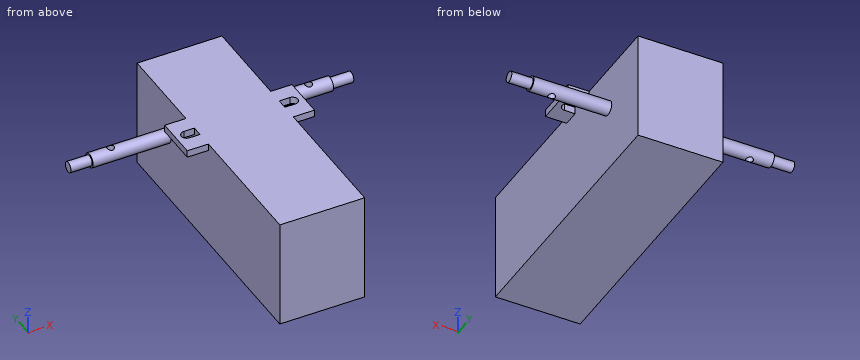
```python
from build123d import *

# Parameters (mm, degrees)
SKETCH1_W                = 24
SKETCH1_H                = 31
BOSS_EXTRUDE1_DEPTH      = 76
BOSS_EXTRUDE2_DEPTH      = 28
BOSS_EXTRUDE2_DEPTH_BACK = 52
SKETCH2_R                = 2
SKETCH7_R                = 2
SKETCH7_R_2              = 1.5
CUT_EXTRUDE1_DEPTH       = 6
SKETCH17_R               = 1
CUT_EXTRUDE3_DEPTH       = 88.271129247
SKETCH18_W               = 2
SKETCH18_H               = 12
BOSS_EXTRUDE3_DEPTH      = 6
CUT_EXTRUDE4_REACH       = 93.307


with BuildPart() as part:
    # Sketch1 → Boss-Extrude1 (new body)
    with BuildSketch(Plane(origin=(0, 0, 0), x_dir=(1, 0, 0), z_dir=(0, 1, 0))):
        Rectangle(SKETCH1_W, SKETCH1_H)
    extrude(amount=BOSS_EXTRUDE1_DEPTH)

    # Sketch2 → Boss-Extrude2 (add, two sides: drawn at the far end of the back side and taken through both)
    with BuildSketch(Plane(origin=(12, 0, 0), x_dir=(0, 0, -1), z_dir=(1, 0, 0)).offset(-BOSS_EXTRUDE2_DEPTH_BACK)):
        with Locations((-3.5, 60)):
            Circle(SKETCH2_R)
    extrude(amount=BOSS_EXTRUDE2_DEPTH + BOSS_EXTRUDE2_DEPTH_BACK)

    # Sketch7 → Cut-Extrude1 (cut)
    with BuildSketch(Plane.ZY.offset(40)):
        with Locations(Location((3.5, 60, 0), (0, 0, 180))):
            Circle(SKETCH7_R)
        with Locations((3.5, 60)):
            Circle(SKETCH7_R_2, mode=Mode.SUBTRACT)
    cut_extrude1 = extrude(amount=-CUT_EXTRUDE1_DEPTH, mode=Mode.SUBTRACT)

    # Sketch17 → Cut-Extrude3 (cut, through all)
    with BuildSketch(Plane.XY):
        with Locations(Location((-28, 60, 0), (0, 0, 180))):
            Circle(SKETCH17_R)
    cut_extrude3 = extrude(amount=CUT_EXTRUDE3_DEPTH, mode=Mode.SUBTRACT)

    # Mirror7: Cut-Extrude1 across plane
    add(cut_extrude1.mirror(Plane(origin=(0, 0, 0), x_dir=(0, 0, 1), z_dir=(1, 0, 0))), mode=Mode.SUBTRACT)

    # Sketch18 → Boss-Extrude3 (add)
    with BuildSketch(Plane(origin=(12, 0, 0), x_dir=(0, 0, -1), z_dir=(1, 0, 0))):
        with Locations((-14.5, 44)):
            Rectangle(SKETCH18_W, SKETCH18_H)
    boss_extrude3 = extrude(amount=BOSS_EXTRUDE3_DEPTH)

    # Sketch19 → Cut-Extrude4 (cut, up to next)
    with BuildSketch(Plane.XY.offset(15.5), mode=Mode.PRIVATE) as cut_extrude4_sk1:
        with BuildLine():
            Line((12, 45.5), (15, 45.5))
            ThreePointArc((15, 45.5), (16.5, 44), (15, 42.5))
            Line((15, 42.5), (12, 42.5))
            Line((12, 42.5), (12, 45.5))
        make_face()
    cut_extrude4_tool1 = extrude(cut_extrude4_sk1.sketch, amount=-CUT_EXTRUDE4_REACH, mode=Mode.PRIVATE) & part.part
    cut_extrude4 = cut_extrude4_tool1.solids().sort_by_distance((14.102462, 44, 15.5))[0]
    add(cut_extrude4, mode=Mode.SUBTRACT)

    # Mirror8: Boss-Extrude3, Cut-Extrude4 across plane
    add(boss_extrude3.mirror(Plane(origin=(0, 0, 0), x_dir=(0, 0, 1), z_dir=(1, 0, 0))))
    add(cut_extrude4.mirror(Plane(origin=(0, 0, 0), x_dir=(0, 0, 1), z_dir=(1, 0, 0))), mode=Mode.SUBTRACT)

    # Mirror9: Cut-Extrude3 across plane
    add(cut_extrude3.mirror(Plane(origin=(0, 0, 0), x_dir=(0, 0, 1), z_dir=(1, 0, 0))), mode=Mode.SUBTRACT)


solid = part.part
```
Model file for the job. Use its own axes, mm. Round coordinates to 2 decimals unless told otherwise and drop trailing zeros. Write each loop counter-clockwise with the first axis right and the second up, starting at its lowest first coordinate (ties: lowest second). Pieces come first, ordered by that corner, then holes. Notation, with made-up numbers: (20, 10.25) - (56, 10.25) arc R20 ccw to (56, 31.25) - close; hole circle Ø11 at (-12, 84). An arc over 180 degrees is marked (long way). Use CSV: the item, a comma, the result in double quotes. Start each with the question number.
Item 1: Drill centre lines: L1, parallel to X at y = 60, z = 3.9; L2, parallel to X at y = 69.5, z = -13; L3, parallel to Y at x = 28, z = 4.65. Where is each one in solid material? Low to high. Write a range as [from, to].
Item 2: Band-saw the part on B-B (z = 3.5). Write the cut outline in (x, y), and give its area (3 significant figures).
Item 3: Band-saw the part on D-D (y = 44). Write the cut outline in (x, z), and give its area (3 significant figures).
Item 4: Pin check, flat tips, straight feed: P1, Ø2.5, axis at x = 28, y = 60, coming from the +Z side; P2, Ø2, axis at x = -14.5, z = 15, coming from the +Y side; P3, Ø1.8, axis at x = -13.5, y = 42.5, coming from the -Z side; P4, Ø6.5, axis at x = 14, y = 46, coming from the -Z side. Stop position of each tip, or through.
Item 5: Band-saw the part on C-C (x = -14). Write the cut outline in (y, z), and give its area (3 significant figures).
Item 6: Band-saw the part on A-A (y = 60). Write the cut outline in (x, z), and give its area (3 significant figures).
Checked values:
1,L1,"x = [-40, -29], [-27, 27], [29, 40]"
1,L2,"x = [-12, 12]"
1,L3,"y = [58.36, 59], [61, 61.64]"
2,outline,"(-40, 58.5) - (-34, 58.5) - (-34, 58) - (-12, 58) - (-12, 0) - (12, 0) - (12, 58) - (34, 58) - (34, 58.5) - (40, 58.5) - (40, 61.5) - (34, 61.5) - (34, 62) - (12, 62) - (12, 76) - (-12, 76) - (-12, 62) - (-34, 62) - (-34, 61.5) - (-40, 61.5) - close; hole circle Ø2 at (-28, 60); hole circle Ø2 at (28, 60)"
2,area,"2,030 mm²"
3,outline,"(-18, 13.5) - (-16.5, 13.5) - (-16.5, 15.5) - (-18, 15.5) - close; (-12, -15.5) - (12, -15.5) - (12, 15.5) - (-12, 15.5) - close; (16.5, 13.5) - (18, 13.5) - (18, 15.5) - (16.5, 15.5) - close"
3,area,"750 mm²"
4,P1,"stops at z = 5.5"
4,P2,"stops at y = 50"
4,P3,"stops at z = 13.5"
4,P4,"stops at z = -15.5"
5,outline,"(38, 13.5) - (42.5, 13.5) - (42.5, 15.5) - (38, 15.5) - close; (45.5, 13.5) - (50, 13.5) - (50, 15.5) - (45.5, 15.5) - close; circle Ø4 at (60, 3.5)"
5,area,"30.6 mm²"
6,outline,"(-40, 2) - (-34, 2) - (-34, 1.5) - (-29, 1.5) - (-29, 5.5) - (-34, 5.5) - (-34, 5) - (-40, 5) - close; (-27, 1.5) - (-12, 1.5) - (-12, -15.5) - (12, -15.5) - (12, 1.5) - (27, 1.5) - (27, 5.5) - (12, 5.5) - (12, 15.5) - (-12, 15.5) - (-12, 5.5) - (-27, 5.5) - close; (29, 1.5) - (34, 1.5) - (34, 2) - (40, 2) - (40, 5) - (34, 5) - (34, 5.5) - (29, 5.5) - close"
6,area,"940 mm²"
